Geometry: see drawing. Coordinates: mm, zero at the bounding-box minimum. A direction names the side the tool comes from. Give positions to 0.01 mm unless a question says otherwise; leave off trailing zeros. Loops run counter-clockwise (first coordinate to the right, second up) from the corner with the lowest first, then second, coordinate; pieces in that order, holes last. Notation, with made-up numbers: (22.25, 49) -> (79.25, 49) arc R23 ccw to (79.25, 75) -> close; hole circle Ø11 at (-37.75, 1.25). An arc over 180 degrees is marked (long way). Return JSON: item names as keys, results as strings. Group by question number.
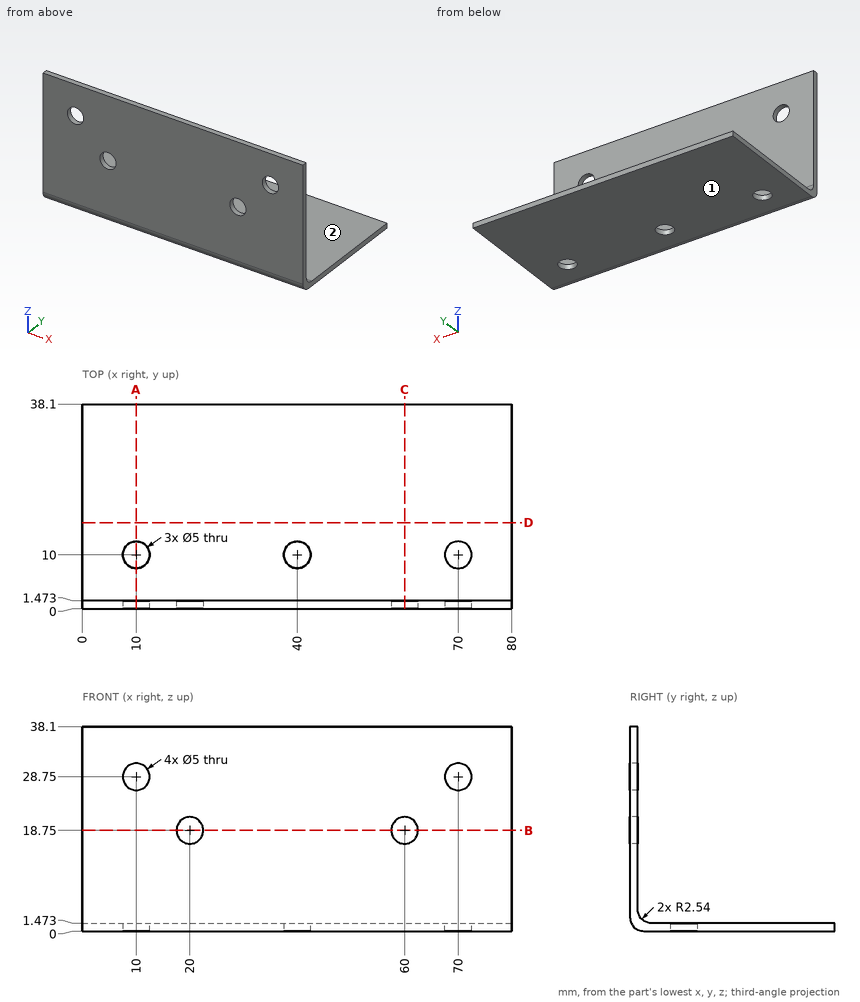
1) Cut plane D-D on y = 16. Return loops of the section in (x, z).
2) Material intervals for line 1 (Z direction, x = 58.5, y = 28.5); line 2 (Z direction, x = 60, y = 1), sorted ascending.
3) Reachability of the marked faces 1 and 2 from +Z, -Z, +X, -X, +Y, -Y: full face, straight path, thin tool, end or side. Return the list, or none.
4) Cut plane C-C on x = 60. Return loops of the section in (y, z), then the cut area to 3 significant figures.
5) Cut plane B-B on z = 18.75. Return loops of the section in (x, y).
6) Cut plane A-A on x = 10. Return loops of the section in (y, z).
7) Contact query for flat-ended pins moving along their axis: P1, Ø4, axis at x = 60, z = 18.75, coming from the +Y side; P2, Ø3, axis at x = 18.5, z = 10.5, coming from the +Y side; P3, Ø3, axis at x = 27.5, y = 28.5, coming from the +Z side. Output: stop coordinate, or through.
Calculated:
{
 "1": {"outline": "(0, 0) -> (80, 0) -> (80, 1.47) -> (0, 1.47) -> close"},
 "2": {"line 1": "0 to 1.47", "line 2": "0.52 to 16.25, 21.25 to 38.1"},
 "3": {"face 1": "-Z, +X, -X, +Y, -Y", "face 2": "+Z, +X, -X, +Y"},
 "4": {"outline": "(0, 2.54) arc R2.54 ccw to (2.54, 0) -> (38.1, 0) -> (38.1, 1.47) -> (4.01, 1.47) arc R2.54 cw to (1.47, 4.01) -> (1.47, 16.25) -> (0, 16.25) -> close; (0, 21.25) -> (1.47, 21.25) -> (1.47, 38.1) -> (0, 38.1) -> close", "area": "103 mm2"},
 "5": {"outline": "(0, 0) -> (17.5, 0) -> (17.5, 1.47) -> (0, 1.47) -> close; (22.5, 0) -> (57.5, 0) -> (57.5, 1.47) -> (22.5, 1.47) -> close; (62.5, 0) -> (80, 0) -> (80, 1.47) -> (62.5, 1.47) -> close"},
 "6": {"outline": "(0, 2.54) arc R2.54 ccw to (2.54, 0) -> (7.5, 0) -> (7.5, 1.47) -> (4.01, 1.47) arc R2.54 cw to (1.47, 4.01) -> (1.47, 26.25) -> (0, 26.25) -> close; (0, 31.25) -> (1.47, 31.25) -> (1.47, 38.1) -> (0, 38.1) -> close; (12.5, 0) -> (38.1, 0) -> (38.1, 1.47) -> (12.5, 1.47) -> close"},
 "7": {"P1": "through", "P2": "y = 1.47", "P3": "z = 1.47"}
}
